Check sheet for the modelled part. Datum: model origin and axes. Units: mm. A direction names the side the tool comes from. Coordinates: 2 decimals unless noted, no trailing zeros. Loops run counter-clockwise (first coordinate to the right, second up) from the corner with the lowest first, then second, coordinate; pieces in that order, holes last. Notation, with made-up numbers: M 75,55 L 113,55 A22 cw 113,88 Z; hole C 44,-30.75 d11. An arc over 180 degrees is marked long. Answer in a Markdown table with one row per item. Add a question column.
```python
from build123d import *

# Parameters (mm, degrees)
F0_R      = 3.48
F1_DEPTH  = 6.88
F3_DEPTH  = 6.881
F5_DEPTH  = 6.89
F6_W      = 5.37
F6_H      = 4.37
F7_DEPTH  = 3.32
F8_R      = 2.4
F9_DEPTH  = 1.93
F10_R     = 2.4
F11_DEPTH = 4.99
F12_R     = 1.12
F13_DEPTH = 6.23


with BuildPart() as f1:
    # F0 (on Front) → F1 (new body)
    with BuildSketch(Plane.XZ):
        Circle(F0_R)
    extrude(amount=F1_DEPTH)

    # F2 (on face) → F3 (cut, through all)
    with BuildSketch(Plane(origin=(0, 0, 0), x_dir=(-1, 0, 0), z_dir=(0, 1, 0))):
        Polygon((4.844351, 2.141895), (3.33, 4.121852), (3.33, -5.87584), align=None)
    extrude(amount=-F3_DEPTH, mode=Mode.SUBTRACT)

    # F4 (on face) → F5 (join)
    with BuildSketch(Plane(origin=(0, 0, 0), x_dir=(-1, 0, 0), z_dir=(0, 1, 0))):
        with BuildLine():
            Line((3.33, -10.320693), (3.33, -1.010693))
            ThreePointArc((3.33, -1.010693), (0.84212, -2.838426), (-2.24, -2.663231))
            Line((-2.24, -2.663231), (-2.24, -6.990693))
            Line((-2.24, -6.990693), (-4.56, -6.990693))
            Line((-4.56, -6.990693), (-4.56, -10.320693))
            Line((-4.56, -10.320693), (3.33, -10.320693))
        make_face()
    extrude(amount=-F5_DEPTH)

    # F6 (on face) → F7 (cut)
    with BuildSketch(Plane(origin=(0, 0, -10.320693), x_dir=(1, 0, 0), z_dir=(0, 0, -1))):
        with Locations((0.615, 3.445)):
            Rectangle(F6_W, F6_H)
    extrude(amount=-F7_DEPTH, mode=Mode.SUBTRACT)

    # F8 (on face) → F9 (cut)
    with BuildSketch(Plane(origin=(-3.33, 0, 0), x_dir=(0, -1, 0), z_dir=(-1, 0, 0))):
        with Locations((3.44, 0)):
            Circle(F8_R)
    extrude(amount=-F9_DEPTH, mode=Mode.SUBTRACT)

    # F10 (on face) → F11 (cut)
    with BuildSketch(Plane(origin=(-3.33, 0, 0), x_dir=(0, -1, 0), z_dir=(-1, 0, 0))):
        with Locations((3.445, -6.270693)):
            Circle(F10_R)
    extrude(amount=-F11_DEPTH, mode=Mode.SUBTRACT)

    # F12 (on face) → F13 (cut)
    with BuildSketch(Plane.XZ.offset(6.88)):
        Circle(F12_R)
    extrude(amount=-F13_DEPTH, mode=Mode.SUBTRACT)


solid = f1.part
```
Q1. Mould release check, pull along Z, two halves, no side actions. Record for faces 4 (the face through (-1.4, -3, 0)), 5 (the face through (1, -1, -10.321)), 6 (the face through (1, -1.26, -9)): released by +Z, released by -Z, zero draft, split by the parting line, or undercut.
Q2. Cross-section at D-D (x = 2.5). Record the cut outline in (y, z), plus the area to 3 significant figures.
Q3. Cross-section at B-B (z = -9). Record the cut outline in (x, y).
Q4. Cross-section at A-A (y = -3.44). Record the cut outline in (x, z), plus the area to 3 significant figures.
Q5. Access from +Z, -Z, +X, -X, +Y, -Y to the whole of each face (thin tool, end or side, straight path). Record for faces 1 (the face through (2, -3, -7.001)), 2 (the face through (-2.07, -3, -9)), 3 (the face through (2.24, -3, -5)).
Q6. Cross-section at C-C (y = -2.25). Record the cut outline in (x, z).
Q7. Go/stop test with flat-tipped pins: pin 1 (2.5 mm diameter, centred on x = 3.5, y = -4.5, fed in from +Z); pin 2 (0.7 mm diameter, centred on x = 0, z = 0, fed in from -Y); pin 3 (1.3 mm diameter, centred on x = 2.5, y = -3.5, fed in from -Z). Record where each tip stops, or that it passes through.
Q8. Thickness scan on L1, parallel to Y at x = 1, z = -7.75; L2, parallel to Z at x = -2.5, y = -4.75; L3, parallel to Y at x = -0.75, z = -4.5. Record the ranges inside material, lowest first.
Answer key:
| question | item | result |
|---|---|---|
| 1 | face 4 | undercut |
| 1 | face 5 | released by -Z |
| 1 | face 6 | zero draft |
| 2 | outline | M -6.89,-10.32 L -5.63,-10.32 L -5.63,-7 L -1.26,-7 L -1.26,-10.32 L 0,-10.32 L 0,-6.99 L -6.89,-6.99 Z; M -6.88,-2.42 L 0,-2.42 L 0,2.42 L -6.88,2.42 Z |
| 2 | area | 41.7 mm^2 |
| 3 | outline | M -3.33,-6.89 L 4.56,-6.89 L 4.56,0 L -3.33,0 Z; hole M -2.07,-5.63 L 3.3,-5.63 L 3.3,-1.26 L -2.07,-1.26 Z |
| 4 | outline | M -3.33,-10.32 L -2.07,-10.32 L -2.07,-8.67 L -3.33,-8.67 Z; M -3.33,-3.87 L 1.66,-3.87 L 1.66,-7 L 3.3,-7 L 3.3,-10.32 L 4.56,-10.32 L 4.56,-6.99 L 2.24,-6.99 L 2.24,-2.66 A3.48 ccw long -2.52,2.4 L -1.4,2.4 L -1.4,-2.4 L -3.33,-2.4 Z; hole C 0,0 d2.24 |
| 4 | area | 38.1 mm^2 |
| 5 | face 1 | -Z, -X |
| 5 | face 2 | -Z |
| 5 | face 3 | +X, +Y, -Y |
| 6 | outline | M -3.33,-10.32 L -2.07,-10.32 L -2.07,-8.35 L -3.33,-8.35 Z; M -3.33,-4.19 L 1.66,-4.19 L 1.66,-7 L 3.3,-7 L 3.3,-10.32 L 4.56,-10.32 L 4.56,-6.99 L 2.24,-6.99 L 2.24,-2.66 A3.48 ccw long -2.79,2.08 L -1.4,2.08 L -1.4,-2.08 L -3.33,-2.08 Z; hole C 0,0 d2.24 |
| 7 | pin 1 | z = 2.65 |
| 7 | pin 2 | y = -0.65 |
| 7 | pin 3 | z = -7 |
| 8 | L1 | -6.89 to -5.63, -1.26 to 0 |
| 8 | L2 | -10.32 to -8.28, -4.26 to -2.01, 2.01 to 2.42 |
| 8 | L3 | -6.89 to -5.07, -1.82 to 0 |
